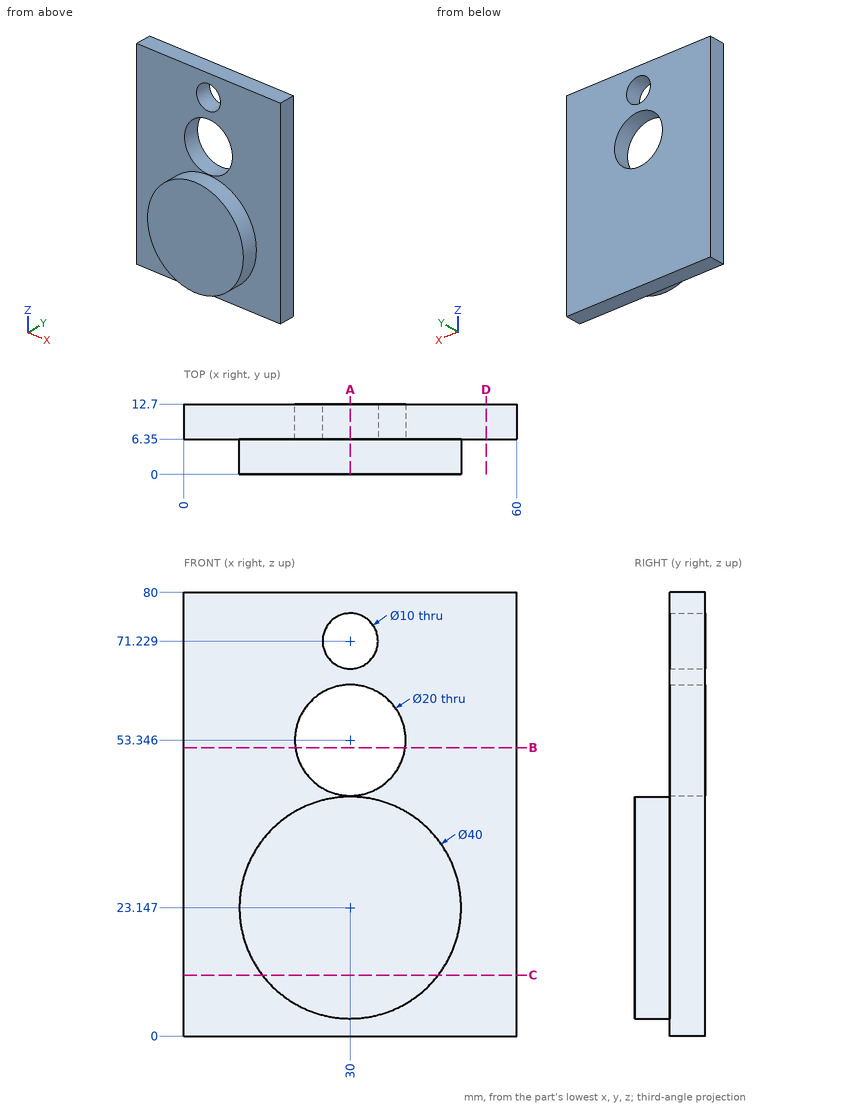
Study the drawing (mm; zero at the part's minimum x, y, z) and answer. Coordinates: 2 decimals unless noted, no trailing zeros. Order: outer loops, then holes, each group sorted by start corner. A loop starts at its lowest first (then second) coordinate and runs counter-clockwise, first axis right, second up. Notation, with made-up numbers: (20, 85.5) -> (45, 85.5) arc R34 ccw to (45, 119.5) -> close; hole circle Ø8 at (0, 44). An arc over 180 degrees is marked (long way). Answer in a Markdown table with one row per item. Add a question column.
Item 1: Find section D-D (x = 54.5). Write down the section's boundary in (y, z).
Item 2: Each of these flat-tipped pins is pushed along its axis until it touches: P1, Ø2, axis at x = 32.5, z = 14, coming from the -Y side; P2, Ø16, axis at x = 30, z = 53.35, coming from the +Y side; P3, Ø3, axis at y = 2, z = 15, coming from the -X side. Where does it stop, or does it pass through?
Item 3: Find section C-C (z = 11). Write down the section's boundary in (x, y), then the cut area to 3 significant figures.
Item 4: Find the intervals of material crossed by L1, parallel to Z at x = 30, y = 7.5; L2, parallel to X at y = 6.5, z = 71.5; L3, parallel to Y at x = 52, z = 23, in increasing order. Write a range as from..to.
Item 5: Find section B-B (z = 52). Write down the section's boundary in (x, y), then the cut area to 3 significant figures.
Item 6: Find section A-A (x = 30). Write down the section's boundary in (y, z).
Result set:
| question | item | result |
|---|---|---|
| 1 | outline | (6.35, 0) -> (12.7, 0) -> (12.7, 80) -> (6.35, 80) -> close |
| 2 | P1 | stops at y = 0 |
| 2 | P2 | passes through |
| 2 | P3 | stops at x = 11.14 |
| 3 | outline | (0, 6.35) -> (14.11, 6.35) -> (14.11, 0) -> (45.89, 0) -> (45.89, 6.35) -> (60, 6.35) -> (60, 12.7) -> (0, 12.7) -> close |
| 3 | area | 583 mm² |
| 4 | L1 | z = 0..43.35, 63.35..66.23, 76.23..80 |
| 4 | L2 | x = 0..25.01, 34.99..60 |
| 4 | L3 | y = 6.35..12.7 |
| 5 | outline | (0, 6.35) -> (20.09, 6.35) -> (20.09, 12.7) -> (0, 12.7) -> close; (39.91, 6.35) -> (60, 6.35) -> (60, 12.7) -> (39.91, 12.7) -> close |
| 5 | area | 255 mm² |
| 6 | outline | (0, 3.15) -> (6.35, 3.15) -> (6.35, 0) -> (12.7, 0) -> (12.7, 43.35) -> (6.35, 43.35) -> (6.35, 43.15) -> (0, 43.15) -> close; (6.35, 63.35) -> (12.7, 63.35) -> (12.7, 66.23) -> (6.35, 66.23) -> close; (6.35, 76.23) -> (12.7, 76.23) -> (12.7, 80) -> (6.35, 80) -> close |
